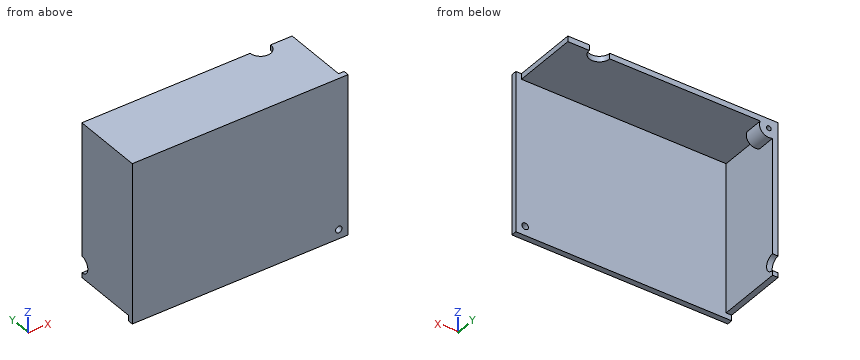
from build123d import *

# Parameters (mm, degrees)
SKETCH1_W           = 116
SKETCH1_H           = 86
BOSS_EXTRUDE1_DEPTH = 3
SKETCH2_W           = 113
SKETCH2_H           = 3
BOSS_EXTRUDE2_DEPTH = 35
SKETCH3_W           = 3
SKETCH3_H           = 80
BOSS_EXTRUDE3_DEPTH = 35
SKETCH4_R           = 1.75
CUT_EXTRUDE1_DEPTH  = 35
SKETCH5_R           = 5
SKETCH5_R_2         = 1.25
BOSS_EXTRUDE4_DEPTH = 10
SKETCH6_R           = 5.5
CUT_EXTRUDE2_DEPTH  = 10
SKETCH7_R           = 4.5
CUT_EXTRUDE3_DEPTH  = 10


with BuildPart() as part:
    # Sketch1 → Boss-Extrude1 (new body)
    with BuildSketch(Plane(origin=(0, 0, 0), x_dir=(1, 0, 0), z_dir=(0, 1, 0))):
        with Locations((58, 43)):
            Rectangle(SKETCH1_W, SKETCH1_H)
    extrude(amount=BOSS_EXTRUDE1_DEPTH)

    # Sketch2 → Boss-Extrude2 (add)
    with BuildSketch(Plane(origin=(0, 3, 0), x_dir=(1, 0, 0), z_dir=(0, 1, 0))):
        with Locations((56.5, 1.5)):
            Rectangle(SKETCH2_W, SKETCH2_H)
    extrude(amount=BOSS_EXTRUDE2_DEPTH)

    # Sketch3 → Boss-Extrude3 (add)
    with BuildSketch(Plane(origin=(0, 3, 0), x_dir=(1, 0, 0), z_dir=(0, 1, 0))):
        with Locations((1.5, 43)):
            Rectangle(SKETCH3_W, SKETCH3_H)
    extrude(amount=BOSS_EXTRUDE3_DEPTH)

    # Sketch4 → Cut-Extrude1 (cut)
    with BuildSketch(Plane.XZ):
        with Locations((111, -81)):
            Circle(SKETCH4_R)
    extrude(amount=-CUT_EXTRUDE1_DEPTH, mode=Mode.SUBTRACT)

    # Sketch5 → Boss-Extrude4 (add)
    with BuildSketch(Plane(origin=(0, 38, 0), x_dir=(1, 0, 0), z_dir=(0, 1, 0))):
        with Locations((5, 5)):
            Circle(SKETCH5_R)
        with Locations((5, 5)):
            Circle(SKETCH5_R_2, mode=Mode.SUBTRACT)
    extrude(amount=-BOSS_EXTRUDE4_DEPTH)

    # Sketch6 → Cut-Extrude2 (cut)
    with BuildSketch(Plane.XY):
        with Locations((96, 38)):
            Circle(SKETCH6_R)
    extrude(amount=-CUT_EXTRUDE2_DEPTH, mode=Mode.SUBTRACT)

    # Sketch7 → Cut-Extrude3 (cut)
    with BuildSketch(Plane.ZY):
        with Locations((-76, 38)):
            Circle(SKETCH7_R)
    extrude(amount=-CUT_EXTRUDE3_DEPTH, mode=Mode.SUBTRACT)


solid = part.part
For this review, take the finished solid that the model builds, in its own axes (mm). Round coordinates to 2 decimals unless told otherwise and drop trailing zeros. Order: outer loops, then holes, each group sorted by start corner. A loop starts at its lowest first (then second) coordinate and runs counter-clockwise, first axis right, second up. Notation, with made-up numbers: M 62.5,75 L 72.5,75 A23 cw 72.5,109 Z; hole C 65,-26 d3. An arc over 180 degrees is marked long. Use a Markdown table: item, result. Add a question column.
Item 1: Add section B-B, the plane x = 5. Give the boundary of the cut face in (y, z), then the cut area to 3 significant figures.
Item 2: Add section A-A, the plane z = -5. Give the boundary of the cut face in (x, y).
Item 3: Add section C-C, the plane z = -76. Give the boundary of the cut face in (x, y), then the cut area to 4 significant figures.
Item 4: Add section D-D, the plane x = 111. Give the boundary of the cut face in (y, z), then the cut area to 4 significant figures.
Item 5: To check wall thickness, follow line 1 along Z through (x, y) = (5, 33.75); line 2 along Z through (x, y) = (111, 1.6); line 3 along X through (y, z) = (35.75, -5). State the ranges of each line that lie inside material, in increasing order.
Item 6: Insertion check: pin 1 (10.5 mm diameter, centred on y = 16.5, z = -54, fed in from +X); pin 2 (1.5 mm diameter, centred on y = 12.5, z = -1.5, fed in from +X); pin 3 (10.5 mm diameter, centred on x = 69.5, y = 19, fed in from -Z). Each pin has a flat end and moves straight along its axis. Give the tip position at first contact, or say it passes through.
Geometry results:
| question | item | result |
|---|---|---|
| 1 | outline | M 0,-86 L 3,-86 L 3,-3 L 28,-3 L 28,-3.75 L 38,-3.75 L 38,0 L 0,0 Z; M 28,-10 L 38,-10 L 38,-6.25 L 28,-6.25 Z |
| 1 | area | 408 mm² |
| 2 | outline | M 0,0 L 116,0 L 116,3 L 3,3 L 3,28 L 3.75,28 L 3.75,38 L 0,38 Z; M 6.25,28 L 10,28 L 10,38 L 6.25,38 Z |
| 3 | outline | M 0,0 L 116,0 L 116,3 L 3,3 L 3,33.5 L 0,33.5 Z |
| 3 | area | 439.5 mm² |
| 4 | outline | M 0,-86 L 3,-86 L 3,-82.75 L 0,-82.75 Z; M 0,-79.25 L 3,-79.25 L 3,-3 L 38,-3 L 38,0 L 0,0 Z |
| 4 | area | 352.5 mm² |
| 5 | line 1 | z = -10 to -6.25, -3.75 to 0 |
| 5 | line 2 | z = -86 to -82.75, -79.25 to 0 |
| 5 | line 3 | x = 0 to 3.75, 6.25 to 10 |
| 6 | pin 1 | stops at x = 3 |
| 6 | pin 2 | stops at x = 113 |
| 6 | pin 3 | stops at z = -3 |
